Design review of the part built by this model. Coordinates are the model's own, in mm. A direction names the side the tool comes from. Give positions to 0.01 mm unless a question says otherwise; leave off trailing zeros. Write each loop counter-clockwise with the first axis right and the second up, starting at its lowest first coordinate (ties: lowest second). Pieces come first, ordered by that corner, then holes. Notation, with made-up numbers: (64.25, -35.5) -> (112.25, -35.5) arc R28 cw to (112.25, -5.5) -> close; hole circle Ø4 at (34, 31.25). An arc over 180 degrees is marked (long way). Answer as a JSON object with one key per item and string values.
```python
from build123d import *
from build123d.topology import SkipClean

# Parameters (mm, degrees)
SKETCH1_W           = 57
SKETCH1_H           = 183.5
SKETCH1_W_2         = 49
SKETCH1_H_2         = 175.5
BOSS_EXTRUDE1_DEPTH = 30
BOSS_EXTRUDE2_DEPTH = 175.5
FILLET1_R           = 14
CUT_EXTRUDE1_DEPTH  = 179.5
SKETCH6_R           = 1.6
SKETCH6_R_2         = 1.45
BOSS_EXTRUDE5_DEPTH = 10


with BuildPart() as part:
    # Sketch1 → Boss-Extrude1 (new body)
    with BuildSketch(Plane.XY):
        with Locations((0, 18.25)):
            Rectangle(SKETCH1_W, SKETCH1_H)
        with Locations((0, 18.25)):
            Rectangle(SKETCH1_W_2, SKETCH1_H_2, mode=Mode.SUBTRACT)
    extrude(amount=BOSS_EXTRUDE1_DEPTH)

    # Sketch2 → Boss-Extrude2 (add)
    with BuildSketch(Plane(origin=(0, -69.5, 0), x_dir=(1, 0, 0), z_dir=(0, 1, 0))):
        with BuildLine():
            Line((14.5, -26), (24.5, -26))
            Line((24.5, -26), (24.5, -16))
            ThreePointArc((24.5, -16), (21.571067812, -23.071067812), (14.5, -26))
        make_face()
        Polygon((-24.5, -30), (24.5, -30), (24.5, -26), (14.5, -26), (-14.5, -26), (-24.5, -26), align=None)
        with BuildLine():
            Line((-24.5, -16), (-24.5, -26))
            Line((-24.5, -26), (-14.5, -26))
            ThreePointArc((-14.5, -26), (-21.571067812, -23.071067812), (-24.5, -16))
        make_face()
    extrude(amount=BOSS_EXTRUDE2_DEPTH)

    # Fillet1
    fillet1_edges = [part.edges().sort_by_distance(p)[0] for p in [
        (-28.5, 18.25, 30),
        (28.5, 18.25, 30),
    ]]
    fillet(fillet1_edges, radius=FILLET1_R)

    # Sketch2<4> → Cut-Extrude1 (cut)
    with SkipClean():  # the faces are left unmerged after this step: merging them gives an invalid solid
        with BuildSketch(Plane(origin=(0, -69.5, 0), x_dir=(1, 0, 0), z_dir=(0, 1, 0))):
            with BuildLine():
                Line((-14.5, -26), (14.5, -26))
                ThreePointArc((14.5, -26), (21.571067812, -23.071067812), (24.5, -16))
                Line((24.5, -16), (24.5, 0))
                Line((24.5, 0), (-24.5, 0))
                Line((-24.5, 0), (-24.5, -16))
                ThreePointArc((-24.5, -16), (-21.571067812, -23.071067812), (-14.5, -26))
            make_face()
        extrude(amount=CUT_EXTRUDE1_DEPTH, mode=Mode.SUBTRACT)
    add(part.part.scale(1), mode=Mode.REPLACE)  # the faces are merged on a copy

    # Sketch6 → Boss-Extrude5 (add)
    # profile 1 of 2: a face of its own
    with BuildSketch(Plane(origin=(0, 110, 0), x_dir=(1, 0, 0), z_dir=(0, 1, 0))):
        with BuildLine():
            ThreePointArc((1, -35.2), (2.13137085, -34.73137085), (2.6, -33.6))
            Line((2.6, -33.6), (2.6, -32))
            ThreePointArc((2.6, -32), (3.185786438, -30.585786438), (4.6, -30))
            Line((4.6, -30), (-4.6, -30))
            ThreePointArc((-4.6, -30), (-3.185786438, -30.585786438), (-2.6, -32))
            Line((-2.6, -32), (-2.6, -33.6))
            ThreePointArc((-2.6, -33.6), (-2.13137085, -34.73137085), (-1, -35.2))
            Line((-1, -35.2), (1, -35.2))
        make_face()
        with Locations((0, -32.8)):
            Circle(SKETCH6_R, mode=Mode.SUBTRACT)
    # profile 2 of 2: a face of its own
    with BuildSketch(Plane(origin=(0, 110, 0), x_dir=(1, 0, 0), z_dir=(0, 1, 0))):
        with Locations((0, -32.8)):
            Circle(SKETCH6_R)
        with Locations(Location((0, -32.8, 0), (0, 0, 270))):
            Circle(SKETCH6_R_2, mode=Mode.SUBTRACT)
    extrude(amount=-BOSS_EXTRUDE5_DEPTH)


solid = part.part
```
(1) The part is to be moulded in two halves that separate along X. For faces 1 (the cylindrical face through (-24.5, 19.5, 25.8)), 2 (the cylindrical face through (21.49, 18.99, 23.15)), 3 (the cylindrical face through (-21.65, 18.99, 22.99)), 4 (the flat face through (0, -73.5, 15)), say which applies: +X half, -X half, draft (parallel to the pull), parting line (faces both ways), or undercut.
Here are the results:
{"face 1": "-X half", "face 2": "undercut", "face 3": "undercut", "face 4": "draft"}
(2) We need section C-C, the plane z = 24. State the section outline as (x, y) points.
Here are the results:
{"outline": "(-25.99, -73.5) -> (25.99, -73.5) -> (25.99, 110) -> (20.5, 110) -> (20.5, -69.5) -> (-20.5, -69.5) -> (-20.5, 110) -> (-25.99, 110) -> close"}
(3) Clearance check with flat-ended pins moving along their axes: pin 1 (2 mm diameter, centred on x = 5.5, y = -51.5, fed in from -Z); pin 2 (6 mm diameter, centred on y = 4, z = 22.5, fed in from +X); pin 3 (1.5 mm diameter, centred on y = 41.5, z = 26, fed in from -X); pin 4 (1.7 mm diameter, centred on x = 0, z = 32.8, fed in from -Y). State where each tip first meets the part, or that it passes through.
Here are the results:
{"pin 1": "stops at z = 26", "pin 2": "stops at x = 28.06", "pin 3": "stops at x = -25.01", "pin 4": "passes through"}
(4) We need section A-A, the plane y = -9. State the section outline as (x, z) points, then the cut area to 3 significant figures.
Here are the results:
{"outline": "(-28.5, 0) -> (-24.5, 0) -> (-24.5, 16) arc R10 cw to (-14.5, 26) -> (14.5, 26) arc R10 cw to (24.5, 16) -> (24.5, 0) -> (28.5, 0) -> (28.5, 16) arc R14 ccw to (14.5, 30) -> (-14.5, 30) arc R14 ccw to (-28.5, 16) -> close", "area": "395 mm²"}
(5) For faces 5 (the flat face through (28.5, 17, 8)), 6 (the flat face through (1, 100, 31)), 7 (the flat face through (-24.5, 19, 8)), list the 3-axis set-ups (+Z, -Z, +X, -X, +Y, -Y) from which the entire face can be reached by the end or side of a thin tool; tool diameter is ignored.
Here are the results:
{"face 5": "+Z, -Z, +X, +Y, -Y", "face 6": "+Z, +X, -X, -Y", "face 7": "-Z, +Y"}
(6) We need section D-D, the plane x = 21.5. State the section outline as (y, z) points.
Here are the results:
{"outline": "(-73.5, 0) -> (-69.5, 0) -> (-69.5, 23.14) -> (110, 23.14) -> (110, 28.12) -> (-73.5, 28.12) -> close"}
(7) For line 1 along X through (y, z) = (-42, 7); line 2 along X through (y, z) = (104.25, 32.8); line 3 along Y through (x, z) = (-17, 10), list the stretches that pass through material, from the lowest coordinate up.
Here are the results:
{"line 1": "x = -28.5 to -24.5, 24.5 to 28.5", "line 2": "x = -2.6 to -1.45, 1.45 to 2.6", "line 3": "y = -73.5 to -69.5"}
(8) We need section B-B, the plane x = 7.5. State the section outline as (y, z) points, then the cut area to 3 significant figures.
Here are the results:
{"outline": "(-73.5, 0) -> (-69.5, 0) -> (-69.5, 26) -> (110, 26) -> (110, 30) -> (-73.5, 30) -> close", "area": "838 mm²"}
